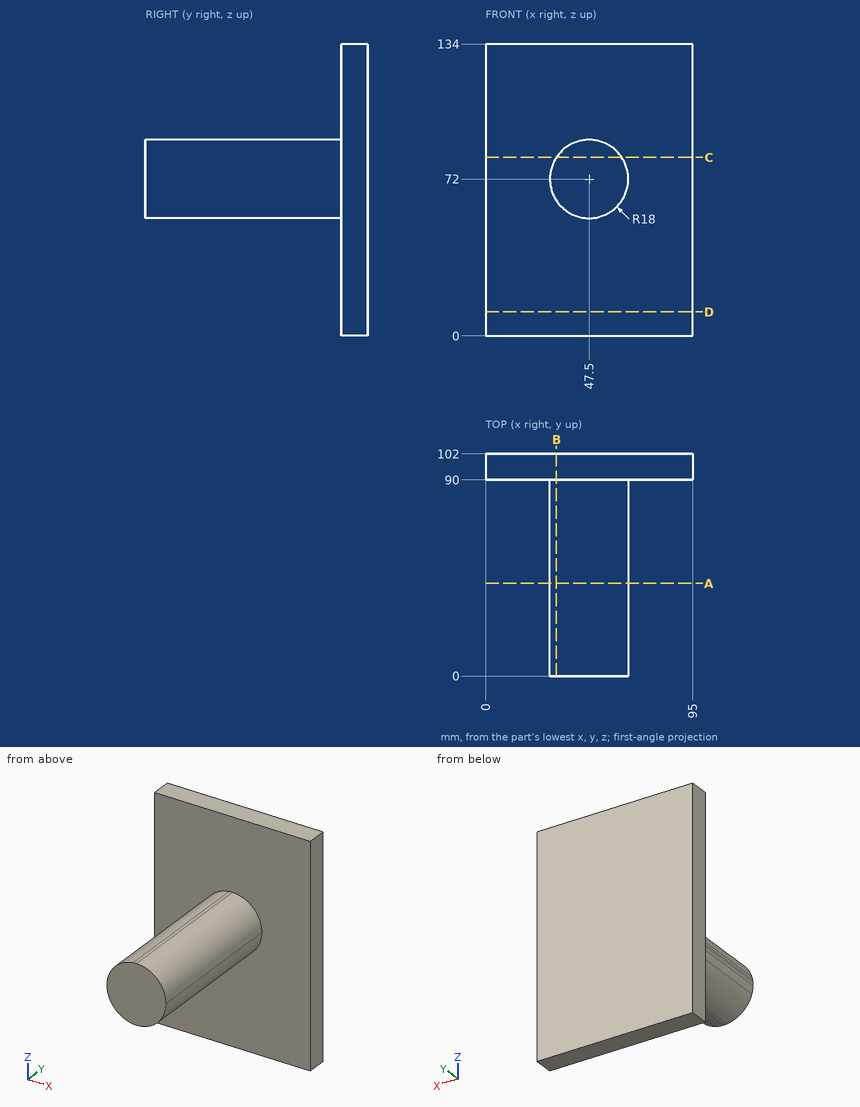
Source: three-view drawing plus pictorial views. Frame: mm from the lowest corner of the part. Coordinates: 2 decimals unless noted, no trailing zeros. Write each loop counter-clockwise with the first axis right and the second up, starting at its lowest first coordinate (ties: lowest second). Pieces come first, ordered by that corner, then holes. Notation, with made-up numbers: (10, 75) -> (46, 75) arc R34 ccw to (46, 112) -> close; hole circle Ø3 at (35, 0). An arc over 180 degrees is marked (long way). Write each question's results on one line, items separated by ' | '.
Item 1: Material intervals for probe 1 along Y at (x, z) = (43, 90.5); probe 2 along Z at (x, y) = (49.5, 73); probe 3 along X at (y, z) = (88, 71.5), sorted ascending.
Conclusion:
probe 1: y = 90 to 102 | probe 2: z = 54.11 to 89.89 | probe 3: x = 29.51 to 65.49
Item 2: Section query C-C on z = 82. Return loops of the section in (x, y).
Conclusion:
outline: (0, 90) -> (32.53, 90) -> (32.53, 0) -> (62.47, 0) -> (62.47, 90) -> (95, 90) -> (95, 102) -> (0, 102) -> close
Item 3: Section query A-A on y = 42.5. Return loops of the section in (x, z), plus the area to 3 significant figures.
Conclusion:
outline: circle Ø36 at (47.5, 72) | area: 1,020 mm^2
Item 4: Section query D-D on z = 11. Return loops of the section in (x, y).
Conclusion:
outline: (0, 90) -> (95, 90) -> (95, 102) -> (0, 102) -> close
Item 5: Pin query (flat end, axial travel): pin 1 Ø10 at (x, z) = (9.5, 63) entering from -Y; pin 2 Ø5 at (x, y) = (52, 54) entering from +Z; pin 3 Ø10 at (x, y) = (30, 77) entering from -Z. Return the tip coordinate at first contact, or that it passes through.
Conclusion:
pin 1: stops at y = 90 | pin 2: stops at z = 89.89 | pin 3: stops at z = 59.05
Item 6: Section query B-B on x = 32.5. Return loops of the section in (y, z).
Conclusion:
outline: (0, 62.05) -> (90, 62.05) -> (90, 0) -> (102, 0) -> (102, 134) -> (90, 134) -> (90, 81.95) -> (0, 81.95) -> close
